```python
from build123d import *

# Parameters (mm, degrees)
BOSS_EXTRUDE1_DEPTH = 38.1
SKETCH2_R           = 3.175
CUT_EXTRUDE1_DEPTH  = 39.1
SKETCH3_R           = 1.4732
CUT_EXTRUDE2_DEPTH  = 13.7


with BuildPart() as part:
    # Sketch1 → Boss-Extrude1 (new body)
    with BuildSketch(Plane(origin=(0, 0, 0), x_dir=(0, 0, -1), z_dir=(1, 0, 0))):
        Polygon((0, 0), (0, 12.7), (12.7, 12.7), (12.7, 76.2), (25.4, 76.2), (25.4, 0), align=None)
    extrude(amount=BOSS_EXTRUDE1_DEPTH)

    # Sketch2 → Cut-Extrude1 (cut, through all)
    with BuildSketch(Plane(origin=(38.1, 0, 0), x_dir=(0, 0, -1), z_dir=(1, 0, 0))):
        with Locations((19.05, 50.8)):
            Circle(SKETCH2_R)
    extrude(amount=-CUT_EXTRUDE1_DEPTH, mode=Mode.SUBTRACT)

    # Sketch3 → Cut-Extrude2 (cut, through all)
    with BuildSketch(Plane(origin=(0, 12.7, 0), x_dir=(1, 0, 0), z_dir=(0, 1, 0))):
        with Locations((9.525, 6.35)):
            Circle(SKETCH3_R)
        with Locations((28.575, 6.35)):
            Circle(SKETCH3_R)
    extrude(amount=-CUT_EXTRUDE2_DEPTH, mode=Mode.SUBTRACT)


solid = part.part
```
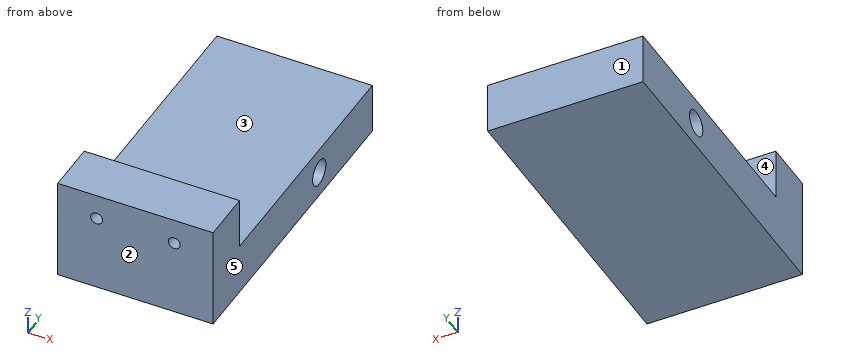
Input: part model. Units: mm. Frame: model coordinates. Face numbers are marked on the shaded views. A direction names the side the tool comes from. Round coordinates to 2 decimals unless told otherwise and drop trailing zeros. Order: outer loops, then holes, each group sorted by start corner. A loop starts at its lowest first (then second) coordinate and runs counter-clockwise, first axis right, second up. Notation, with made-up numbers: (56.25, 24) - (107.25, 24) arc R31 ccw to (107.25, 53) - close; hole circle Ø10 at (60, 67). An arc over 180 degrees is marked (long way). One line per question, with ' | ' between items. Start each with the question number.
1) Cut plane C-C, the plane y = 50.8. Return the cut outline in (x, z) (3 decimals), then the cut area to 3 significant figures.
2) Cut plane A-A, the plane x = 4.5. Return the cut outline in (y, z) (3 decimals), then the cut area to 3 significant figures.
3) Contact query for flat-ended pins moving along their axis: P1, Ø12, axis at x = 15, y = 22, coming from the +Z side; P2, Ø4.5, axis at x = 28.575, z = -6.35, coming from the -Y side. Output: stop coordinate, or through.
4) Cut plane D-D, the plane x = 9. Return the cut outline in (y, z) (3 decimals).
5) Ray query, probe 1 along X at (y, z) = (7.5, -6.35); probe 2 along Z at (x, y) = (5, 24); probe 3 along Y at (x, z) = (8, -4.75). Return the intervals inside material, ascending.
6) Cut plane B-B, the plane z = -19.05. Return the cut outline in (x, y) (3 decimals).
7) Set-up query: the marked faces 4 and 5. Return all of +Z, -Z, +X, -X, +Y, -Y with unobstructed straight access to the full face (end or side cutting, diameter ignored); none if empty.
8) Pull-direction query (Y, two-part tool) for the marked faces 1, 2 and 3; classes: +Y half, -Y half, draft (parallel to the pull), parting line (faces both ways), or undercut.
Worked out:
1) outline: (0, -25.4) - (38.1, -25.4) - (38.1, -22.225) - (0, -22.225) - close; (0, -15.875) - (38.1, -15.875) - (38.1, -12.7) - (0, -12.7) - close | area: 242 mm^2
2) outline: (0, -25.4) - (76.2, -25.4) - (76.2, -12.7) - (12.7, -12.7) - (12.7, 0) - (0, 0) - close; hole circle Ø6.35 at (50.8, -19.05) | area: 1,100 mm^2
3) P1: stops at z = -12.7 | P2: stops at y = 0
4) outline: (0, -25.4) - (76.2, -25.4) - (76.2, -12.7) - (12.7, -12.7) - (12.7, -7.726) - (0, -7.726) - close; (0, -4.974) - (12.7, -4.974) - (12.7, 0) - (0, 0) - close; hole circle Ø6.35 at (50.8, -19.05)
5) probe 1: x = 0 to 8.05, 11 to 27.1, 30.05 to 38.1 | probe 2: z = -25.4 to -12.7 | probe 3: y = 0 to 12.7
6) outline: (0, 0) - (38.1, 0) - (38.1, 47.625) - (0, 47.625) - close; (0, 53.975) - (38.1, 53.975) - (38.1, 76.2) - (0, 76.2) - close
7) face 4: +Z, +X, -X, +Y | face 5: +Z, -Z, +X, +Y, -Y
8) face 1: +Y half | face 2: -Y half | face 3: draft
